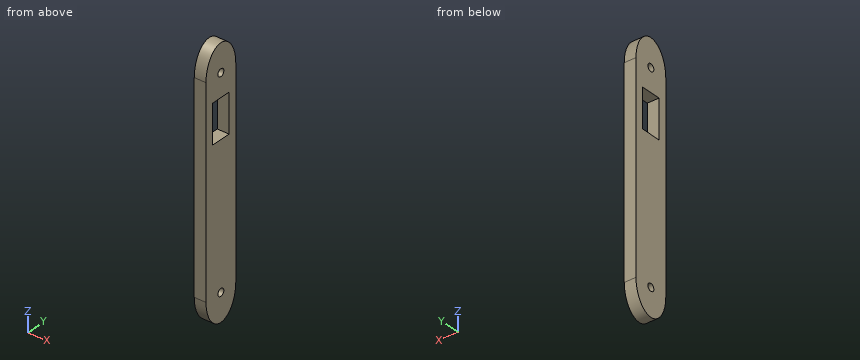
from build123d import *

# Parameters (mm, degrees)
SKETCH1_RX          = 30
SKETCH1_RY          = 20
SKETCH1_W           = 220
SKETCH1_H           = 40
BOSS_EXTRUDE1_DEPTH = 12.7
SKETCH2_R           = 4
SKETCH2_W           = 42
SKETCH2_H           = 22
CUT_EXTRUDE1_DEPTH  = 12.7


with BuildPart() as part:
    # Sketch1 → Boss-Extrude1 (new body)
    with BuildSketch(Plane(origin=(0, 0, 0), x_dir=(0, 0, -1), z_dir=(1, 0, 0))):
        with Locations(Location((-110, 0), (0, 0, 0))):
            Ellipse(SKETCH1_RX, SKETCH1_RY)
        with Locations(Location((110, 0), (0, 0, -180))):
            Ellipse(SKETCH1_RX, SKETCH1_RY)
        Rectangle(SKETCH1_W, SKETCH1_H)
    extrude(amount=BOSS_EXTRUDE1_DEPTH)

    # Sketch2 → Cut-Extrude1 (cut)
    with BuildSketch(Plane(origin=(12.7, 0, 0), x_dir=(0, 0, -1), z_dir=(1, 0, 0))):
        with Locations((-110, 0)):
            Circle(SKETCH2_R)
        with Locations(Location((110, 0, 0), (0, 0, 180))):
            Circle(SKETCH2_R)
        with Locations((-64, 0)):
            Rectangle(SKETCH2_W, SKETCH2_H)
    extrude(amount=-CUT_EXTRUDE1_DEPTH, mode=Mode.SUBTRACT)


solid = part.part
Geometry check sheet. Reference: the model listing, model coordinates, mm. Coordinates: 2 decimals unless noted, no trailing zeros. Order: outer loops, then holes, each group sorted by start corner. A loop starts at its lowest first (then second) coordinate and runs counter-clockwise, first axis right, second up. Notation, with made-up numbers: (28, 56.25) - (61, 56.25) arc R29 cw to (61, 79.25) - close; hole circle Ø8 at (-35, 22). An arc over 180 degrees is marked (long way). One line per item, written item: value.
(1) Depth check by flat-ended pin: pin 1 Ø6.5 at (x, y) = (9, 5) entering from -Z; pin 2 Ø7 at (y, z) = (0, -110) entering from -X; pin 3 Ø1 at (x, y) = (5.5, 3.5) entering from -Z. Enter the tip coordinate at first touch or a pass-through.
Data:
pin 1: stops at z = -139.88
pin 2: passes through
pin 3: stops at z = -139.66
(2) Sectioned sample at A-A (z = 59). Enter the section's corners in (x, y).
Data:
outline: (0, -20) - (12.7, -20) - (12.7, -11) - (0, -11) - close; (0, 11) - (12.7, 11) - (12.7, 20) - (0, 20) - close
(3) Sectioned sample at B-B (y = 0). Count the separate pieces of the cut face and the enclosed holes in it, and give its area (3 significant figures).
Data:
separate pieces: 4
enclosed holes: 0
area: 2,820 mm^2
(4) Thickness scan on probe 1 along Y at (x, z) = (7.5, 110); probe 2 along Y at (x, z) = (7, 49); probe 3 along Z at (x, y) = (9.25, 10.5). Record the ranges inside material, lowest first. Write a range as from..to.
Data:
probe 1: y = -20..-4, 4..20
probe 2: y = -20..-11, 11..20
probe 3: z = -135.53..43, 85..135.53
